Autodesk Inventor part; units mm, degrees
ref_plane "YZ Plane" through (0, 0, 0) normal (1, 0, 0) x (0, 1, 0)
ref_plane "XZ Plane" through (0, 0, 0) normal (0, 1, 0) x (-1, 0, 0)
ref_plane "XY Plane" through (0, 0, 0) normal (0, 0, 1) x (1, 0, 0)
sketch "Sketch1" plane through (0, 0, 0) normal (0, 1, 0) x (-1, 0, 0)
  line L0 (35, 107.75) -> (-35, 107.75)
  line L1 (-35, 107.75) -> (-35, -107.75)
  line L2 (-35, -107.75) -> (35, -107.75)
  line L3 (35, -107.75) -> (35, 107.75)
  line L4 (35, 107.75) -> (-35, -107.75) construction
  line L5 (-35, 107.75) -> (35, -107.75) construction
  circle A0 centre (30, -102.75) radius 1.5
  circle A1 centre (-30, -102.75) radius 1.5
  point P0 (0, 0)
  dimension "d0" = 70
  dimension "d1" = 215.5
  dimension "d2" = 3
  dimension "d3" = 3
  dimension "d4" = 5
  dimension "d5" = 5
  dimension "d6" = 5
  dimension "d7" = 5
extrude "Extrusion1" add sketch "Sketch1" along normal blind 1
sketch "Sketch2" plane through (0, 1, 0) normal (0, 1, 0) x (1, 0, 0)
  line L0 (-35, -107.75) -> (35, -107.75)
  line L1 (-35, -107.75) -> (-25, -107.75)
  line L2 (-25, -107.75) -> (-25, -57.75)
  line L3 (-25, -57.75) -> (-35, -57.75)
  line L4 (-35, -57.75) -> (-35, -107.75)
  line L5 (35, -107.75) -> (25, -107.75)
  line L6 (25, -107.75) -> (25, -57.75)
  line L7 (25, -57.75) -> (35, -57.75)
  line L8 (35, -57.75) -> (35, -107.75)
  line L9 (-25, -107.75) -> (-35, -57.75)
  line L10 (25, -107.75) -> (35, -57.75)
  point P0 (0, 0)
  dimension "d10" = 10
  dimension "d11" = 50
  dimension "d12" = 10
  dimension "d13" = 50
extrude "Extrusion2" cut sketch "Sketch2" against normal up to next contours L4 L9 L0 | L10 L8 L0
sketch "Sketch3" plane through (0, 1, 0) normal (0, 1, 0) x (1, 0, 0)
  circle A0 centre (-30, -2.25) radius 1.5
  circle A1 centre (30, -2.25) radius 1.5
  line L0 (-25, -107.75) -> (25, -107.75)
  line L1 (-35, 107.75) -> (-35, -57.75)
  line L2 (35, -57.75) -> (35, 107.75)
  circle A2 centre (0, -102.75) radius 1.5
  point P0 (0, 0)
  dimension "d16" = 3
  dimension "d17" = 3
  dimension "d18" = 105.5
  dimension "d19" = 105.5
  dimension "d20" = 5
  dimension "d21" = 5
  dimension "d22" = 3
  dimension "d23" = 5
extrude "Extrusion3" cut sketch "Sketch3" against normal up to next
properties part number "cover2" material "PET Plastic"
Check sheet for the modelled part. Datum: model origin and axes. Units: mm. Give positions to 0.01 mm unless a question says otherwise; leave off trailing zeros. Loops run counter-clockwise (first coordinate to the right, second up) from the corner with the lowest first, then second, coordinate; pieces in that order, holes last. Notation, with made-up numbers: M 3,48 L 50,48 A19 ccw 50,69 Z; hole C 10,79 d9. An arc over 180 degrees is marked long. Use a Markdown table: item, result. Add a question column.
Q1. Sectioned sample at A-A, the plane y = 0.75. Record the cut outline in (x, z), then the cut area to 3 significant figures.
Q2. Go/stop test with a flat-tipped pin: pin 1 (2.5 mm diameter, centred on x = 30, z = -102.75, fed in from -Y). Record where the tip stops, or that it passes through.
Q3. Scan lines: line 1 along X through (y, z) = (0.5, -102.75); line 2 along X through (y, z) = (0.65, 102.75); line 3 along X through (y, z) = (0.4, 92). Record each from-to range of solid material in increasing order. Write a range as [from, to].
Q4. Sectioned sample at B-B, the plane z = 71. Record the cut outline in (x, y), then the cut area to 3 significant figures.
Verdict:
| question | item | result |
|---|---|---|
| 1 | outline | M -35,-107.75 L 35,-107.75 L 35,57.75 L 25,107.75 L -25,107.75 L -35,57.75 Z; hole C -30,-102.75 d3; hole C -30,2.25 d3; hole C 0,102.75 d3; hole C 30,-102.75 d3; hole C 30,2.25 d3 |
| 1 | area | 14,500 mm^2 |
| 2 | pin 1 | through |
| 3 | line 1 | [-35, -31.5], [-28.5, 28.5], [31.5, 35] |
| 3 | line 2 | [-26, -1.5], [1.5, 26] |
| 3 | line 3 | [-28.15, 28.15] |
| 4 | outline | M -32.35,0 L 32.35,0 L 32.35,1 L -32.35,1 Z |
| 4 | area | 64.7 mm^2 |
